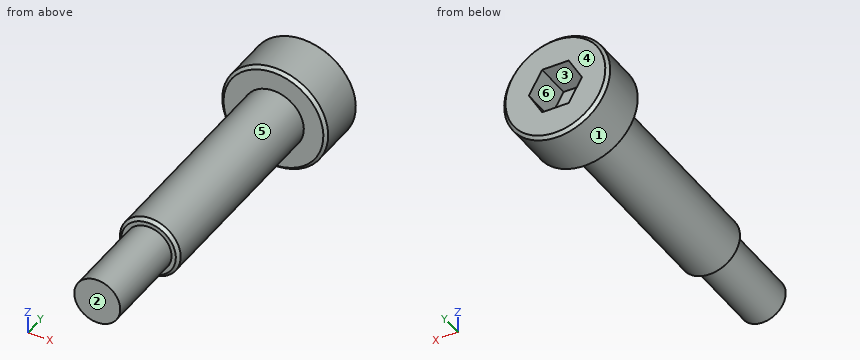
from build123d import *

# Parameters (mm, degrees)
CUT_EXTRUDE1_DEPTH = 2.4
CHAMFER1_SIZE      = 0.2


with BuildPart() as part:
    # Sketch1 → Revolve1 (revolve)
    with BuildSketch(Plane.XY, mode=Mode.PRIVATE) as revolve1_sk:
        Polygon((0, 0), (1.5, 0), (1.5, 5.75), (1.98, 5.75), (1.98, 19.75), (3.455, 19.75), (3.455, 23.24), (0, 23.24), align=None)
    revolve(revolve1_sk.sketch.rotate(Axis((0, 23.24, 0), (0, -1, 0)), 90), axis=Axis((0, 23.24, 0), (0, -1, 0)))

    # Sketch2 → Cut-Extrude1 (cut)
    with BuildSketch(Plane(origin=(0, 23.24, 0), x_dir=(1, 0, 0), z_dir=(0, 1, 0))):
        Polygon((1.732050808, 0), (0.866025404, 1.5), (-0.866025404, 1.5), (-1.732050808, 0), (-0.866025404, -1.5), (0.866025404, -1.5), align=None)
    extrude(amount=-CUT_EXTRUDE1_DEPTH, mode=Mode.SUBTRACT)

    # Chamfer1
    chamfer1_edges = [part.edges().sort_by_distance(p)[0] for p in [
        (0, 23.24, -3.455),
        (0, 19.75, -3.455),
        (0, 5.75, -1.98),
    ]]
    chamfer(chamfer1_edges, length=CHAMFER1_SIZE)


solid = part.part
CAD build for the part. Positions are in the model's coordinates, mm. Face numbers are marked on the shaded views. A direction names the side the tool comes from. Round coordinates to 2 decimals unless told otherwise and drop trailing zeros. Write each loop counter-clockwise with the first axis right and the second up, starting at its lowest first coordinate (ties: lowest second). Pieces come first, ordered by that corner, then holes. Notation, with made-up numbers: M 76.25,76 L 130.25,76 A32 ccw 130.25,103 Z; hole C 13,-14.5 d5. An arc over 180 degrees is marked long. Use a Markdown table: item, result. Add a question column.
1. Slice it at C-C on y = 10.75. Give the cut face in (x, z), then the cut area to 3 significant figures.
2. Slice it at A-A on x = 0. Give the cut face in (y, z) (3 decimals), then the cut area to 3 significant figures.
3. Slice it at B-B on y = 5.5. Give the cut face in (x, z).
4. Pull direction X, two halves, no side cores. Call the marked faces 1, 2 and 3: released by +X, released by -X, zero draft, split by the parting line, or undercut.
5. Drill centre lines: probe 1 along Y at (x, z) = (-2, -2.5); probe 2 along Y at (x, z) = (0.75, -1); probe 3 along Z at (x, y) = (-1, 22). Where is each one in solid material? Low to high.
6. 3-axis set-ups, long thin cutter, end or side, ignore diameter. For the marked faces 4, 5 and 6: which of +Z, -Z, +X, -X, +Y, -Y reach the whole face in a straight line?
7. Flat gauge pins, fed straight in: P1, Ø2, axis at x = 0, y = 7, coming from the -Z side; P2, Ø2, axis at x = -2, y = 15.5, coming from the -Z side; P3, Ø2, axis at x = -0.5, y = 19, coming from the -Z side; P4, Ø3, axis at x = 0.5, z = 0.5, coming from the -Y side. Where does each tip first touch, or does it go through?
Reply:
| question | item | result |
|---|---|---|
| 1 | outline | C 0,0 d3.96 |
| 1 | area | 12.3 mm^2 |
| 2 | outline | M 0,-1.5 L 5.75,-1.5 L 5.75,-1.78 L 5.95,-1.98 L 19.75,-1.98 L 19.75,-3.255 L 19.95,-3.455 L 23.04,-3.455 L 23.24,-3.255 L 23.24,-1.5 L 20.84,-1.5 L 20.84,1.5 L 23.24,1.5 L 23.24,3.255 L 23.04,3.455 L 19.95,3.455 L 19.75,3.255 L 19.75,1.98 L 5.95,1.98 L 5.75,1.78 L 5.75,1.5 L 0,1.5 Z |
| 2 | area | 89.5 mm^2 |
| 3 | outline | C 0,0 d3 |
| 4 | face 1 | split by the parting line |
| 4 | face 2 | zero draft |
| 4 | face 3 | undercut |
| 5 | probe 1 | y = 19.75 to 23.24 |
| 5 | probe 2 | y = 0 to 20.84 |
| 5 | probe 3 | z = -3.31 to -1.27, 1.27 to 3.31 |
| 6 | face 4 | +Z, -Z, +X, -X, +Y |
| 6 | face 5 | -Y |
| 6 | face 6 | +Y |
| 7 | P1 | stops at z = -1.98 |
| 7 | P2 | stops at z = -1.71 |
| 7 | P3 | stops at z = -3.45 |
| 7 | P4 | stops at y = 0 |
